from build123d import *

# Parameters (mm, degrees)
SKETCH_1_R      = 2.75
SKETCH_1_R_2    = 1.5
EXTRUDE_1_DEPTH = 6.5
EXTRUDE_START   = 1.5
SKETCH_2_R      = 2
SKETCH_2_R_2    = 1.5
EXTRUDE_2_DEPTH = 1.5
EXTRUDE_START_2 = 5
SKETCH_3_R      = 2.75
SKETCH_3_R_2    = 1.5
EXTRUDE_3_DEPTH = 5
SKETCH_4_R      = 2
SKETCH_4_R_2    = 1.5
EXTRUDE_4_DEPTH = 1.5
SKETCH_5_R      = 2.75
SKETCH_5_R_2    = 1.5
EXTRUDE_5_DEPTH = 5


with BuildPart() as part:
    # 草图1 → 凸台-拉伸1 (new body)
    with BuildSketch(Plane(origin=(0, 0, 0), x_dir=(1, 0, 0), z_dir=(0, 1, 0))):
        with Locations(Location((0, 0, 0), (0, 0, 90))):
            Circle(SKETCH_1_R)
        with Locations(Location((0, 0, 0), (0, 0, 90))):
            Circle(SKETCH_1_R_2, mode=Mode.SUBTRACT)
    extrude(amount=EXTRUDE_1_DEPTH)

    # 草图2 → 凸台-拉伸2 (add)
    with BuildSketch(Plane.XZ.offset(EXTRUDE_START)):
        with Locations(Location((0, 0, 0), (0, 0, 90))):
            Circle(SKETCH_2_R)
        with Locations(Location((0, 0, 0), (0, 0, 270))):
            Circle(SKETCH_2_R_2, mode=Mode.SUBTRACT)
    extrude(amount=-EXTRUDE_2_DEPTH)

    # 草图3 → 凸台-拉伸3 (add)
    with BuildSketch(Plane.XZ.offset(1.5).offset(EXTRUDE_START_2)):
        with Locations(Location((0, 0, 0), (0, 0, 270))):
            Circle(SKETCH_3_R)
        with Locations(Location((0, 0, 0), (0, 0, 270))):
            Circle(SKETCH_3_R_2, mode=Mode.SUBTRACT)
    extrude(amount=-EXTRUDE_3_DEPTH)

    # 草图4 → 凸台-拉伸4 (add)
    with BuildSketch(Plane.XZ.offset(6.5).offset(EXTRUDE_START)):
        with Locations(Location((0, 0, 0), (0, 0, 90))):
            Circle(SKETCH_4_R)
        with Locations(Location((0, 0, 0), (0, 0, 270))):
            Circle(SKETCH_4_R_2, mode=Mode.SUBTRACT)
    extrude(amount=-EXTRUDE_4_DEPTH)

    # 草图5 → 凸台-拉伸5 (add)
    with BuildSketch(Plane.XZ.offset(8).offset(EXTRUDE_START_2)):
        with Locations(Location((0, 0, 0), (0, 0, 270))):
            Circle(SKETCH_5_R)
        with Locations(Location((0, 0, 0), (0, 0, 270))):
            Circle(SKETCH_5_R_2, mode=Mode.SUBTRACT)
    extrude(amount=-EXTRUDE_5_DEPTH)


solid = part.part
Read the model definition and answer for the solid it produces. Units are mm, in the model's axes. A direction names the side the tool comes from. Coordinates: 2 decimals unless noted, no trailing zeros. Write each loop counter-clockwise with the first axis right and the second up, starting at its lowest first coordinate (ties: lowest second). Pieces come first, ordered by that corner, then holes. Notation, with made-up numbers: (-9.75, 33.25) -> (6.25, 33.25) arc R9 cw to (6.25, 42.25) -> close; hole circle Ø7 at (-9, 41.25). An arc over 180 degrees is marked (long way). Return JSON: item names as keys, results as strings.
(1) The part is cut by section B-B on z = 0. Give the vertices of the cut face in (x, y), then the cut area to 4 significant figures.
Answers below:
{"outline": "(-2.75, -13) -> (-1.5, -13) -> (-1.5, 6.5) -> (-2.75, 6.5) -> (-2.75, 0) -> (-2, 0) -> (-2, -1.5) -> (-2.75, -1.5) -> (-2.75, -6.5) -> (-2, -6.5) -> (-2, -8) -> (-2.75, -8) -> close; (1.5, -13) -> (2.75, -13) -> (2.75, -8) -> (2, -8) -> (2, -6.5) -> (2.75, -6.5) -> (2.75, -1.5) -> (2, -1.5) -> (2, 0) -> (2.75, 0) -> (2.75, 6.5) -> (1.5, 6.5) -> close", "area": "44.25 mm^2"}
(2) Consider line 1 along Y through (x, z) = (1.3, 2.3); line 2 along X through (y, z) = (-0.65, 0); line 3 along X through (y, z) = (-9.5, 0). Determine where each line is inside the solid, lowest interval first. Write a range as from..to.
Answers below:
{"line 1": "-13..-8, -6.5..-1.5, 0..6.5", "line 2": "-2..-1.5, 1.5..2", "line 3": "-2.75..-1.5, 1.5..2.75"}
(3) The part is cut by section C-C on x = 2.3. Give the vertices of the cut face in (y, z), then the cut area to 3 significant figures.
Answers below:
{"outline": "(-13, -1.51) -> (-8, -1.51) -> (-8, 1.51) -> (-13, 1.51) -> close; (-6.5, -1.51) -> (-1.5, -1.51) -> (-1.5, 1.51) -> (-6.5, 1.51) -> close; (0, -1.51) -> (6.5, -1.51) -> (6.5, 1.51) -> (0, 1.51) -> close", "area": "49.7 mm^2"}
(4) The part is cut by section D-D on y = -7.25. Give the vertices of the cut face in (x, z).
Answers below:
{"outline": "circle Ø4 at (0, 0); hole circle Ø3 at (0, 0)"}
(5) Which of the six approach directions +Z, -Z, +X, -X, +Y, -Y give full straight-line access (tool end or side, diameter ignored) to faces 1 (the cylindrical face through (-2.685, -4.035, 0.596)), 2 (the cylindrical face through (2, -1, 0))?
Answers below:
{"face 1": "+Y, -Y", "face 2": "none"}
(6) Each of these flat-tipped pins is pushed along its axis until it touches: P1, Ø1.8, axis at x = 0, z = 0, coming from the -Y side; P2, Ø2, axis at y = -8, z = -2, coming from the +X side. Where does it stop, or does it pass through?
Answers below:
{"P1": "through", "P2": "x = 2.56"}
(7) The part is cut by section A-A on x = 0. Give the vertices of the cut face in (y, z), then the cut area to 4 significant figures.
Answers below:
{"outline": "(-13, -2.75) -> (-8, -2.75) -> (-8, -2) -> (-6.5, -2) -> (-6.5, -2.75) -> (-1.5, -2.75) -> (-1.5, -2) -> (0, -2) -> (0, -2.75) -> (6.5, -2.75) -> (6.5, -1.5) -> (-13, -1.5) -> close; (-13, 1.5) -> (6.5, 1.5) -> (6.5, 2.75) -> (0, 2.75) -> (0, 2) -> (-1.5, 2) -> (-1.5, 2.75) -> (-6.5, 2.75) -> (-6.5, 2) -> (-8, 2) -> (-8, 2.75) -> (-13, 2.75) -> close", "area": "44.25 mm^2"}
